The model under review builds one solid part; all positions refer to its coordinate system, in mm. A direction names the side the tool comes from. Give positions to 0.01 mm unless a question says otherwise; leave off trailing zeros. Loops run counter-clockwise (first coordinate to the right, second up) from the corner with the lowest first, then second, coordinate; pieces in that order, holes last. Notation, with made-up numbers: M 68,72.25 L 92,72.25 A10 cw 92,88.25 Z; hole C 29.5,59 d2. An arc over 180 degrees is marked long. Put each result on its own line as item: value. Start each with the question number.
from build123d import *

# Parameters (mm, degrees)
SKETCH2_R               = 40
HOUSING_DEPTH           = 40
SKETCH11_R              = 30
EXTERNALCUT_DEPTH       = 35
INTERNALCUT_START       = -5
SKETCH12_R              = 35
INTERNALCUT_DEPTH       = 30
SKETCH18_W              = 27.94
SKETCH18_H              = 52.97706376
ESP32_DEPTH             = 9.74
SKETCH19_R              = 6
BUZZERINTERNALCUT_DEPTH = 2
SKETCH20_R              = 0.35
BUZZEREXTRENALCUT_DEPTH = 4
SKETCH22_W              = 4.6
SKETCH22_H              = 6.1
BTNITERNALCUT_DEPTH     = 2
SKETCH25_R              = 1.5
BTNEXTRERNALCUT_DEPTH   = 4
SKETCH26_W              = 3.7
SKETCH26_H              = 8.5
CUT_EXTRUDE6_DEPTH      = 2
SKETCH28_W              = 1.7
SKETCH28_H              = 3.6
CUT_EXTRUDE7_DEPTH      = 4


with BuildPart() as part:
    # Sketch2 → Housing (new body)
    with BuildSketch(Plane(origin=(0, 0, 0), x_dir=(1, 0, 0), z_dir=(0, 1, 0))):
        Circle(SKETCH2_R)
    extrude(amount=HOUSING_DEPTH)

    # Sketch11 → ExternalCUt (cut)
    with BuildSketch(Plane(origin=(0, 40, 0), x_dir=(1, 0, 0), z_dir=(0, 1, 0))):
        Circle(SKETCH11_R)
    extrude(amount=-EXTERNALCUT_DEPTH, mode=Mode.SUBTRACT)

    # Sketch12 → InternalCut (cut)
    with BuildSketch(Plane.XZ.offset(INTERNALCUT_START)):
        Circle(SKETCH12_R)
    extrude(amount=-INTERNALCUT_DEPTH, mode=Mode.SUBTRACT)

    # Sketch18 → ESP32 (add)
    with BuildSketch(Plane(origin=(0, 5, 0), x_dir=(1, 0, 0), z_dir=(0, 1, 0))):
        with Locations((0.343820119, 3.916007291)):
            Rectangle(SKETCH18_W, SKETCH18_H)
    extrude(amount=ESP32_DEPTH)

    # Sketch19 → BuzzerInternalCut (cut)
    with BuildSketch(Plane(origin=(0, 5, 0), x_dir=(1, 0, 0), z_dir=(0, 1, 0))):
        with Locations((-25.006618322, 0)):
            Circle(SKETCH19_R)
    extrude(amount=-BUZZERINTERNALCUT_DEPTH, mode=Mode.SUBTRACT)

    # Sketch20 → BuzzerExtrenalCut (cut, through all)
    with BuildSketch(Plane(origin=(0, 3, 0), x_dir=(1, 0, 0), z_dir=(0, 1, 0))):
        with Locations((-24.042348329, 4.522315504)):
            Circle(SKETCH20_R)
        with Locations((-26.042348329, 3.020429056)):
            Circle(SKETCH20_R)
        with Locations((-28.042348329, 3.020429056)):
            Circle(SKETCH20_R)
        with Locations((-30.042348329, 1.518542609)):
            Circle(SKETCH20_R)
        with Locations((-30.042348329, 0.016656161)):
            Circle(SKETCH20_R)
        with Locations((-30.042348329, -1.485230286)):
            Circle(SKETCH20_R)
        with Locations((-28.042348329, 0.016656161)):
            Circle(SKETCH20_R)
        with Locations((-28.042348329, 1.518542609)):
            Circle(SKETCH20_R)
        with Locations((-28.042348329, -1.485230286)):
            Circle(SKETCH20_R)
        with Locations((-28.042348329, -2.987116733)):
            Circle(SKETCH20_R)
        with Locations((-26.042348329, 0.016656161)):
            Circle(SKETCH20_R)
        with Locations((-26.042348329, 1.518542609)):
            Circle(SKETCH20_R)
        with Locations((-26.042348329, -1.485230286)):
            Circle(SKETCH20_R)
        with Locations((-26.042348329, -2.987116733)):
            Circle(SKETCH20_R)
        with Locations((-26.042348329, -4.489003181)):
            Circle(SKETCH20_R)
        with Locations((-24.042348329, -4.489003181)):
            Circle(SKETCH20_R)
        with Locations((-24.042348329, -2.987116733)):
            Circle(SKETCH20_R)
        with Locations((-24.042348329, -1.485230286)):
            Circle(SKETCH20_R)
        with Locations((-24.042348329, 0.016656161)):
            Circle(SKETCH20_R)
        with Locations((-24.042348329, 1.518542609)):
            Circle(SKETCH20_R)
        with Locations((-24.042348329, 3.020429056)):
            Circle(SKETCH20_R)
        with Locations((-22.042348329, 3.020429056)):
            Circle(SKETCH20_R)
        with Locations((-22.042348329, 1.518542609)):
            Circle(SKETCH20_R)
        with Locations((-22.042348329, 0.016656161)):
            Circle(SKETCH20_R)
        with Locations((-22.042348329, -1.485230286)):
            Circle(SKETCH20_R)
        with Locations((-22.042348329, -2.987116733)):
            Circle(SKETCH20_R)
        with Locations((-20.042348329, -1.485230286)):
            Circle(SKETCH20_R)
        with Locations((-20.042348329, 0.016656161)):
            Circle(SKETCH20_R)
        with Locations((-20.042348329, 1.518542609)):
            Circle(SKETCH20_R)
        with Locations((-26.042348329, 4.522315504)):
            Circle(SKETCH20_R)
    extrude(amount=-BUZZEREXTRENALCUT_DEPTH, mode=Mode.SUBTRACT)

    # Sketch22 → BtnIternalCut (cut)
    with BuildSketch(Plane(origin=(0, 5, 0), x_dir=(1, 0, 0), z_dir=(0, 1, 0))):
        with Locations((23.28859565, -11.93832654)):
            Rectangle(SKETCH22_W, SKETCH22_H)
    extrude(amount=-BTNITERNALCUT_DEPTH, mode=Mode.SUBTRACT)

    # Sketch25 → BtnExtrernalCut (cut, through all)
    with BuildSketch(Plane(origin=(0, 3, 0), x_dir=(1, 0, 0), z_dir=(0, 1, 0))):
        with Locations((23.28859565, -11.93832654)):
            Circle(SKETCH25_R)
    extrude(amount=-BTNEXTRERNALCUT_DEPTH, mode=Mode.SUBTRACT)

    # Sketch26 → Cut-Extrude6 (cut)
    with BuildSketch(Plane(origin=(0, 5, 0), x_dir=(1, 0, 0), z_dir=(0, 1, 0))):
        with Locations((23.409044431, 13.599064282)):
            Rectangle(SKETCH26_W, SKETCH26_H)
    extrude(amount=-CUT_EXTRUDE6_DEPTH, mode=Mode.SUBTRACT)

    # Sketch28 → Cut-Extrude7 (cut, through all)
    with BuildSketch(Plane(origin=(0, 3, 0), x_dir=(1, 0, 0), z_dir=(0, 1, 0))):
        with Locations((23.409044431, 13.599064282)):
            Rectangle(SKETCH28_W, SKETCH28_H)
    extrude(amount=-CUT_EXTRUDE7_DEPTH, mode=Mode.SUBTRACT)


solid = part.part
(1) We need section D-D, the plane z = 25.5. Write out the cut boundary in (x, y).
(2) Draft analysis for pull direction Y (two halves, no side actions). For faces 5 (the flat face through (25.589, 4, 12)), 6 (the flat face through (26, 35, 16)), 7 (the flat face through (-1, 0, -1)), state which applies: +Y half, -Y half, draft (parallel to the pull), parting line (faces both ways), or undercut.
(3) We need section B-B, the plane x = 0. Write out the cut boundary in (y, z), plus the area to 3 significant figures.
(4) To check wall thickness, follow L1, parallel to Y at x = 26, z = -22; L2, parallel to X at y = 10, z = -26; L3, parallel to X at y = 6, z = 16. State the ranges of each line that lie inside material, in increasing order. Write a range as [from, to].
(5) Insertion check: pin 1 (1.5 mm diameter, centred on y = 1, z = -13, fed in from +X); pin 2 (3 mm diameter, centred on y = 8.5, z = -3.5, fed in from +X); pin 3 (1 mm diameter, centred on x = 23.5, y = 4, fed in from +Z). Each pin has a flat end and moves straight along its axis. Give the tip position at first contact, or say it passes through.
(6) For faces 1 (the flat face through (22.559, 2, -14)), 2 (the flat face through (0, 10, -30.405)), 3 (the flat face through (23, 4, 8.888)), 4 (the flat face through (6, 40, -30)), list the 3-axis set-ups (+Z, -Z, +X, -X, +Y, -Y) from which the entire face can be reached by the end or side of a thin tool; tool diameter is ignored.
(7) We need section C-C, the plane y = 32. Write out the cut boundary in (x, z), plus the area to 3 significant figures.
(8) We need section A-A, the plane y = 6.5. Write out the cut boundary in (x, z).
Check sheet entries:
1. outline: M -30.82,0 L 30.82,0 L 30.82,40 L 15.8,40 L 15.8,35 L 23.97,35 L 23.97,5 L -23.97,5 L -23.97,35 L -15.8,35 L -15.8,40 L -30.82,40 Z
2. face 5: draft
2. face 6: undercut
2. face 7: -Y half
3. outline: M 0,-40 L 40,-40 L 40,-30 L 35,-30 L 35,-35 L 5,-35 L 5,-30.4 L 14.74,-30.4 L 14.74,22.57 L 5,22.57 L 5,35 L 35,35 L 35,30 L 40,30 L 40,40 L 0,40 Z
3. area: 1,320 mm²
4. L1: y = [0, 5], [35, 40]
4. L2: x = [-30.4, -23.43], [-13.63, 14.31], [23.43, 30.4]
4. L3: x = [-36.66, -31.13], [-13.63, 14.31], [31.13, 36.66]
5. pin 1: stops at x = 38.08
5. pin 2: stops at x = 39.95
5. pin 3: stops at z = 32.73
6. face 1: +Y, -Y
6. face 2: none
6. face 3: +Y
6. face 4: +Z, -Z, +X, -X, +Y
7. outline: C 0,0 d80; hole C 0,0 d70
7. area: 1,180 mm²
8. outline: C 0,0 d80; M -13.63,-30.4 L 14.31,-30.4 L 14.31,22.57 L -13.63,22.57 Z; hole C 0,0 d70
